Can you work these out from the model? Positions are in its coordinate system, mm. A direction names the side the tool comes from. Give positions to 0.01 mm unless a question says otherwise; leave off trailing zeros. Loops run counter-clockwise (first coordinate to the right, second up) from the corner with the lowest first, then second, coordinate; pieces in that order, holes last.
from build123d import *

# Parameters (mm, degrees)
BOSS_EXTRUDE2_DEPTH = 25
SHELL1_START        = 5
SHELL1_OUTLINE_W    = 16
SHELL1_OUTLINE_H    = 15
SHELL1_DEPTH        = 15
FILLET1_R           = 2
FILLET3_R           = 2


# Read off the part's stored shape, not the designer's step: Shell1
with BuildPart() as part:
    # Sketch1 → Boss-Extrude2 (new body)
    with BuildSketch(Plane.XY):
        Polygon((0, 0), (0, 20), (5, 20), (20, 5), (20, 0), align=None)
    extrude(amount=-BOSS_EXTRUDE2_DEPTH)

    # Shell1 outline → Shell1 (cut)
    with BuildSketch(Plane(origin=(0, 0, 0), x_dir=(1, 0, 0), z_dir=(0, 1, 0)).offset(SHELL1_START)):
        with Locations((13, 12.5)):
            Rectangle(SHELL1_OUTLINE_W, SHELL1_OUTLINE_H)
    extrude(amount=SHELL1_DEPTH, mode=Mode.SUBTRACT)

    # Fillet1
    fillet1_edges = [part.edges().sort_by_distance(p)[0] for p in [
        (12.5, 5, -20),
        (5, 12.5, -20),
        (5, 5, -12.5),
        (12.5, 5, -5),
        (5, 12.5, -5),
    ]]
    fillet(fillet1_edges, radius=FILLET1_R)

    # Fillet3
    fillet3_edges = [part.edges().sort_by_distance(p)[0] for p in [
        (2.5, 20, -25),
        (2.5, 20, 0),
        (20, 2.5, 0),
        (20, 2.5, -25),
        (0, 20, -12.5),
        (20, 0, -12.5),
    ]]
    fillet(fillet3_edges, radius=FILLET3_R)


solid = part.part
(1) Suppose I cut it at B-B on y = 11.25. List the corners of the cut face in (x, z) for me.
Returned:
outline: (0, -25) - (13.75, -25) - (13.75, -20) - (7, -20) arc R2 cw to (5, -18) - (5, -7) arc R2 cw to (7, -5) - (13.75, -5) - (13.75, 0) - (0, 0) - close
(2) Which directions (+Z, -Z, +X, -X, +Y, -Y) give clear straight access to the entire face, cutting with the end or side of a thin tool? Please do faces 1 (the cylindrical face through (19.2, 3.5, -24.6)), 2 (the cylindrical face through (13.59, 5.57, -5.6)).
Returned:
face 1: -Z, +X, +Y, -Y
face 2: +X, +Y
(3) Please list where these lines run through material, in increasing order: probe 1 along Z at (x, y) = (11.75, 11.25); probe 2 along X at (y, z) = (7.5, -15).
Returned:
probe 1: z = -25 to -20, -5 to 0
probe 2: x = 0 to 5
(4) Thinking about a two-plate mould opening in X: for faces 3 (the cylindrical face through (5.57, 13.59, -5.6)), 4 (the flat face through (0, 9, -12)), 5 (the flat face through (7, 7, -25)), which applies, pulls with the +X half, pulls with the -X half, needs draft (parallel to the pull), parting line crosses it, or undercut?
Returned:
face 3: pulls with the +X half
face 4: pulls with the -X half
face 5: needs draft
(5) Suppose I cut it at A-A on x = 11.5. List the corners of the cut face in (y, z) for me, plus the area to 3 significant figures.
Returned:
outline: (0, -25) - (13.5, -25) - (13.5, -20) - (7, -20) arc R2 cw to (5, -18) - (5, -7) arc R2 cw to (7, -5) - (13.5, -5) - (13.5, 0) - (0, 0) - close
area: 212 mm2
(6) Suppose I cut it at D-D on z = -3. List the corners of the cut face in (x, y) for me.
Returned:
outline: (0, 0) - (18, 0) arc R2 ccw to (20, 2) - (20, 5) - (5, 20) - (2, 20) arc R2 ccw to (0, 18) - close
(7) Will these pins go through, and if not, where does the flat tip stop? P1, Ø5.5, axis at x = 11.5, y = 14, coming from the -Z side; P2, Ø1.5, axis at y = 11, z = -10.5, coming from the +X side; P3, Ø4, axis at y = 11.5, z = -22, coming from the +X side; P4, Ø8, axis at x = 13, z = -15, coming from the +Y side.
Returned:
P1: stops at z = -25
P2: stops at x = 5
P3: stops at x = 15.5
P4: stops at y = 5.27
(8) Suppose I cut it at C-C on z = -15.5. List the corners of the cut face in (x, y) for me, plus the area to 3 significant figures.
Returned:
outline: (0, 0) - (18, 0) arc R2 ccw to (20, 2) - (20, 5) - (7, 5) arc R2 cw to (5, 7) - (5, 20) - (2, 20) arc R2 ccw to (0, 18) - close
area: 174 mm2
